from build123d import *

# Parameters (mm, degrees)
SKETCH1_R               = 33.85
BOSS_EXTRUDE1_DEPTH     = 12.5
SKETCH2_R               = 2.5
CUT_EXTRUDE1_DEPTH      = 34.85
CUT_EXTRUDE1_DEPTH_BACK = 34.85
SKETCH3_R               = 2.5
CUT_EXTRUDE2_DEPTH      = 34.8500001
CUT_EXTRUDE2_DEPTH_BACK = 34.8500001
SKETCH4_R               = 42.35
BOSS_EXTRUDE2_DEPTH     = 2
SKETCH5_R               = 42.35
SKETCH5_R_2             = 33.85
BOSS_EXTRUDE3_DEPTH     = 150
SKETCH6_R               = 39.35
CUT_EXTRUDE3_DEPTH      = 5


with BuildPart() as part:
    # Sketch1 → Boss-Extrude1 (new body)
    with BuildSketch(Plane(origin=(0, 0, 0), x_dir=(1, 0, 0), z_dir=(0, 1, 0))):
        Circle(SKETCH1_R)
    extrude(amount=BOSS_EXTRUDE1_DEPTH)

    # Sketch2 → Cut-Extrude1 (cut, two sides)
    with BuildSketch(Plane(origin=(0, 0, 0), x_dir=(0, 0, -1), z_dir=(1, 0, 0))) as cut_extrude1_sk:
        with Locations((0, 5)):
            Circle(SKETCH2_R)
    extrude(amount=CUT_EXTRUDE1_DEPTH, mode=Mode.SUBTRACT)
    extrude(cut_extrude1_sk.sketch, amount=-CUT_EXTRUDE1_DEPTH_BACK, mode=Mode.SUBTRACT)

    # Sketch3 → Cut-Extrude2 (cut, two sides)
    with BuildSketch(Plane.XY) as cut_extrude2_sk:
        with Locations((0, 5)):
            Circle(SKETCH3_R)
    extrude(amount=CUT_EXTRUDE2_DEPTH, mode=Mode.SUBTRACT)
    extrude(cut_extrude2_sk.sketch, amount=-CUT_EXTRUDE2_DEPTH_BACK, mode=Mode.SUBTRACT)

    # Sketch4 → Boss-Extrude2 (add)
    with BuildSketch(Plane(origin=(0, 12.5, 0), x_dir=(1, 0, 0), z_dir=(0, 1, 0))):
        Circle(SKETCH4_R)
    extrude(amount=BOSS_EXTRUDE2_DEPTH)

    # Sketch5 → Boss-Extrude3 (add)
    with BuildSketch(Plane(origin=(0, 14.5, 0), x_dir=(1, 0, 0), z_dir=(0, 1, 0))):
        Circle(SKETCH5_R)
        Circle(SKETCH5_R_2, mode=Mode.SUBTRACT)
    extrude(amount=BOSS_EXTRUDE3_DEPTH)

    # Sketch6 → Cut-Extrude3 (cut)
    with BuildSketch(Plane(origin=(0, 164.5, 0), x_dir=(1, 0, 0), z_dir=(0, 1, 0))):
        Circle(SKETCH6_R)
    extrude(amount=-CUT_EXTRUDE3_DEPTH, mode=Mode.SUBTRACT)


solid = part.part
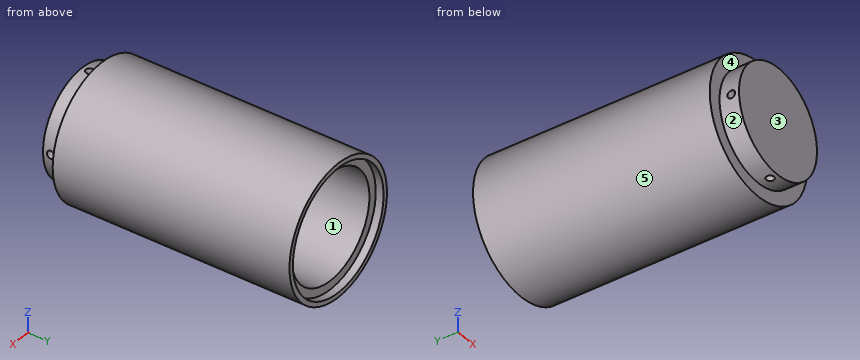
Geometry: final body of the model. Coordinates: model frame, mm. Face numbers are marked on the shaded views. A direction names the side the tool comes from. Coordinates: 2 decimals unless noted, no trailing zeros. Loops run counter-clockwise (first coordinate to the right, second up) from the corner with the lowest first, then second, coordinate; pieces in that order, holes last. Notation, with made-up numbers: M 79.5,-7.5 L 136.5,-7.5 A18 cw 136.5,0.5 Z; hole C 26,79.25 d8. An arc over 180 degrees is marked long. One line per item, written item: value. Start each with the question number.
1) Cut plane B-B (z = 25). Return loops of the section in (x, y).
2) Cut plane C-C (x = 13). Return loops of the section in (y, z), then the cut area to 3 significant figures.
3) Reachability of the marked faces 4 and 5 from +Z, -Z, +X, -X, +Y, -Y: full face, straight path, thin tool, end or side. Return the list, or none.
4) Cut plane D-D (y = 42.5). Return loops of the section in (x, z), then the cut area to 3 significant figures.
5) Cut plane A-A (y = 5). Return loops of the section in (x, z).
6) Draft query along X for the marked faces 1, 2 and 3. Return one class per face: released by +X, released by -X, zero draft, split by the parting line, or undercut.
7) Material intervals for L1, parallel to X at y = 162, z = 0; L2, parallel to X at y = 125, z = 0; L3, parallel to Y at x = -24, z = 0, sorted ascending. Write a range as from..to.
8) Pin query (flat end, axial travel): P1, Ø12, axis at x = -3, y = 85.5, coming from the -Z side; P2, Ø20.5, axis at x = 11.5, z = 3.5, coming from the +Y side; P3, Ø5, axis at y = 62, z = -4, coming from the +X side; P4, Ø2, axis at x = 26, z = 20, coming from the -Y side. Return the tip coordinate at first contact, or that it passes through.
Evaluation:
1. outline: M -34.18,12.5 L -22.82,12.5 L -22.82,0 L 22.82,0 L 22.82,12.5 L 34.18,12.5 L 34.18,164.5 L 30.39,164.5 L 30.39,159.5 L 22.82,159.5 L 22.82,14.5 L -22.82,14.5 L -22.82,159.5 L -30.39,159.5 L -30.39,164.5 L -34.18,164.5 Z; hole C 0,5 d5
2. outline: M 0,-31.25 L 12.5,-31.25 L 12.5,-40.31 L 164.5,-40.31 L 164.5,-37.14 L 159.5,-37.14 L 159.5,-31.25 L 14.5,-31.25 L 14.5,31.25 L 159.5,31.25 L 159.5,37.14 L 164.5,37.14 L 164.5,40.31 L 12.5,40.31 L 12.5,31.25 L 0,31.25 Z; hole C 5,0 d5
2. area: 3,580 mm^2
3. face 4: -Y
3. face 5: +Y, -Y
4. outline: C 0,0 d84.7; hole C 0,0 d67.7
4. area: 2,030 mm^2
5. outline: M -33.76,-2.5 A33.85 ccw -2.5,-33.76 L -2.5,-2.5 Z; M -33.76,2.5 L -2.5,2.5 L -2.5,33.76 A33.85 ccw Z; M 2.5,-33.76 A33.85 ccw 33.76,-2.5 L 2.5,-2.5 Z; M 2.5,2.5 L 33.76,2.5 A33.85 ccw 2.5,33.76 Z
6. face 1: undercut
6. face 2: split by the parting line
6. face 3: zero draft
7. L1: -42.35..-39.35, 39.35..42.35
7. L2: -42.35..-33.85, 33.85..42.35
7. L3: 0..2.5, 7.5..14.5
8. P1: z = -42.35
8. P2: y = 14.5
8. P3: x = 42.32
8. P4: y = 0
